Autodesk Inventor part; units mm, degrees
ref_plane "YZ Plane" through (0, 0, 0) normal (1, 0, 0) x (0, 1, 0)
ref_plane "XZ Plane" through (0, 0, 0) normal (0, 1, 0) x (-1, 0, 0)
ref_plane "XY Plane" through (0, 0, 0) normal (0, 0, 1) x (1, 0, 0)
sketch "Sketch1" plane through (0, 0, 0) normal (0, 1, 0) x (-1, 0, 0)
  line L0 (12.827, 12.827) -> (-12.827, 12.827)
  line L1 (-12.827, 12.827) -> (-12.827, -12.827)
  line L2 (-12.827, -12.827) -> (12.827, -12.827)
  line L3 (12.827, -12.827) -> (12.827, 12.827)
  line L4 (12.827, 12.827) -> (-12.827, -12.827) construction
  line L5 (-12.827, 12.827) -> (12.827, -12.827) construction
  line L6 (16.002, 16.002) -> (-16.002, 16.002)
  line L7 (-16.002, 16.002) -> (-16.002, -16.002)
  line L8 (-16.002, -16.002) -> (16.002, -16.002)
  line L9 (16.002, -16.002) -> (16.002, 16.002)
  point P0 (0, 0)
  dimension "d0" = 25.654
  dimension "d1" = 25.654
  dimension "d2" = 3.175
extrude "Extrusion1" add sketch "Sketch1" along normal blind 50.8
sketch "Sketch2" plane through (16.002, 0, 16.002) normal (1, 0, 0) x (0, 0, -1)
  line L0 (0, 50.8) -> (32.004, 50.8)
  point P0 (16.002, 0)
  point P1 (16.002, 12.7)
  point P2 (16.002, 38.1)
  point P3 (16.002, 50.8)
  dimension "d5" = 12.7
  dimension "d6" = 25.4
hole "Hole1" at (16.002, 12.7, 0) at (16.002, 38.1, 0) direction (-1, 0, 0) diameter 4.445 end through all
sketch "Sketch3" plane through (-16.002, 0, 16.002) normal (0, 0, 1) x (1, 0, 0)
  line L0 (0, 50.8) -> (32.004, 50.8)
  point P0 (16.002, 0)
  point P1 (16.002, 12.7)
  point P2 (16.002, 38.1)
  point P3 (32.004, 38.1)
  point P4 (32.004, 12.7)
  point P5 (16.002, 50.8)
hole "Hole2" at (0, 38.1, 16.002) at (0, 12.7, 16.002) direction (0, 0, -1) diameter 4.445 end through all
sketch "Sketch4" plane through (16.002, 0, 16.002) normal (1, 0, 0) x (0, 0, -1)
  circle A0 centre (16.002, 12.7) radius 2.2225
  circle A1 centre (16.002, 12.7) radius 12.7
  circle A2 centre (16.002, 12.7) radius 16.002
  line L0 (32.004, 0) -> (32.004, 50.8)
  line L1 (0, 0) -> (32.004, 0)
  line L2 (0, 0) -> (0, 50.8)
  circle A3 centre (16.002, 12.7) radius 2.2225
  circle A4 centre (16.002, 12.7) radius 12.827
  point P0 (16.002, 0)
  point P1 (0, 12.7)
  point P2 (32.004, 12.7)
  point P3 (14.201464, 0)
  point P4 (17.802536, 0)
  dimension "d26" = 25.4
  dimension "d27" = 25.654
extrude "Extrusion2" add sketch "Sketch4" along normal blind 34.925 contours L1 A2 A4 | L1 L2 A2 | A2 L0 L1 picked at (30.667502, 14.995372)
sketch "Sketch4 outline for Extrusion3" plane through (16.002, 0, 16.002) normal (1, 0, 0) x (0, 0, -1)
  circle A0 centre (16.002, 12.7) radius 2.2225
  arc A1 (17.802536, 0) -> (14.201464, 0) centre (16.002, 12.7) ccw
  line L0 (14.201464, 0) -> (17.802536, 0)
extrude "Extrusion3" cut sketch "Sketch4 outline for Extrusion3" against normal up to surface (28.829 mm away)
fillet "Fillet1" radius 6.35 1 edges at (16.002, 28.702, 0)
properties part number "Tracking Wheel Guide"
Design review of the part built by this model. Coordinates are the model's own, in mm. A direction names the side the tool comes from. Round coordinates to 2 decimals unless told otherwise and drop trailing zeros. Order: outer loops, then holes, each group sorted by start corner. A loop starts at its lowest first (then second) coordinate and runs counter-clockwise, first axis right, second up.
1) Draft analysis for pull direction X (two halves, no side actions). For faces 1 (the cylindrical face through (36.44, 28.7, 0.35)), 2 (the flat face through (-16.002, 25, 0)), 3 (the cylindrical face through (0.851, 36.047, -14.437)), state which applies: released by +X, released by -X, zero draft, split by the parting line, or undercut.
The answers:
face 1: zero draft
face 2: released by -X
face 3: undercut
2) Consider section D-D (y = 45.5). State the section outline as (x, z) points.
The answers:
outline: (-16, -16) - (16, -16) - (16, 16) - (-16, 16) - close; hole (-12.83, -12.83) - (12.83, -12.83) - (12.83, 12.83) - (-12.83, 12.83) - close
3) Consider section C-C (y = 38.1). State the section outline as (x, z) points, plus the area to 3 significant figures.
The answers:
outline: (-16, -16) - (-2.22, -16) - (-2.22, -12.83) - (-12.83, -12.83) - (-12.83, -2.22) - (-16, -2.22) - close; (-16, 2.22) - (-12.83, 2.22) - (-12.83, 12.83) - (-2.22, 12.83) - (-2.22, 16) - (-16, 16) - close; (2.22, -16) - (16, -16) - (16, -2.22) - (12.83, -2.22) - (12.83, -12.83) - (2.22, -12.83) - close; (2.22, 12.83) - (12.83, 12.83) - (12.83, 2.22) - (16, 2.22) - (16, 16) - (2.22, 16) - close
area: 310 mm2
4) Clearance check with flat-ended pins moving along their axes: pin 1 Ø3 at (x, y) = (33.5, 24) entering from +Z; pin 2 Ø2 at (x, z) = (38, -8) entering from +Y; pin 3 Ø4 at (x, z) = (43.5, -6) entering from +Y. State where each tip first meets the part, or that it passes through.
The answers:
pin 1: stops at z = 12.65
pin 2: stops at y = 27.09
pin 3: stops at y = 28.19
5) Consider section A-A (x = 10.5). State the section outline as (y, z) points, plus the area to 3 significant figures.
The answers:
outline: (0, -16) - (50.8, -16) - (50.8, -12.83) - (0, -12.83) - close; (0, 12.83) - (50.8, 12.83) - (50.8, 16) - (0, 16) - close
area: 323 mm2
6) Consider section B-B (z = 0). State the section outline as (x, y) points.
The answers:
outline: (-16, 0) - (-12.83, 0) - (-12.83, 10.48) - (-16, 10.48) - close; (-16, 14.92) - (-12.83, 14.92) - (-12.83, 35.88) - (-16, 35.88) - close; (-16, 40.32) - (-12.83, 40.32) - (-12.83, 50.8) - (-16, 50.8) - close; (12.83, 25.53) - (50.93, 25.53) - (50.93, 28.7) - (22.35, 28.7) arc R6.35 cw to (16, 35.05) - (16, 35.88) - (12.83, 35.88) - close; (12.83, 40.32) - (16, 40.32) - (16, 50.8) - (12.83, 50.8) - close
7) For L1, parallel to Y at x = 0, z = -14.55; L2, parallel to Z at x = -10, y = 33.5; L3, parallel to X at y = 38, z = -13, list the stretches that pass through material, from the lowest coordinate up.
The answers:
L1: y = 0 to 10.48, 14.92 to 35.88, 40.32 to 50.8
L2: z = -16 to -12.83, 12.83 to 16
L3: x = -16 to -2.22, 2.22 to 16
8) Machinability: for faces 4 (the flat face through (12.827, 3, 10)), 5 (the cylindrical face through (32.144, 25.516, -0.539)), 6 (the cylindrical face through (-14.437, 10.496, 0.289)), which of the approach directions +Z, -Z, +X, -X, +Y, -Y give a long, thin tool a straight path to every point of the face, cutting with its end or side? Answer none if there is none.
The answers:
face 4: +Y, -Y
face 5: +X
face 6: +X, -X
